Geometry check sheet. Reference: the model listing, model coordinates, mm. Face numbers are marked on the shaded views. A direction names the side the tool comes from. Coordinates: 2 decimals unless noted, no trailing zeros. Order: outer loops, then holes, each group sorted by start corner. A loop starts at its lowest first (then second) coordinate and runs counter-clockwise, first axis right, second up. Notation, with made-up numbers: (70, -39.5) - (100, -39.5) arc R34 ccw to (100, -1.5) - close; hole circle Ø5 at (-27, 22.5). An arc over 180 degrees is marked (long way). Use CSV: the item, a comma, the result in double quotes. Start each with the question number.
1) Sectioned sample at B-B, the plane z = 48. Record the cut outline in (x, y), and give its area (3 significant figures).
2) Thickness scan on probe 1 along X at (y, z) = (-7.25, 23.5); probe 2 along Z at (x, y) = (42, -3); probe 3 along Y at (x, z) = (40, -50). Record the ranges inside material, lowest first. Write a range as [from, to].
3) Tool access check on the marked faces 5 and 6. Record the directions out of +Z, -Z, +X, -X, +Y, -Y that give a thin tool (end or side, any length) a straight path to the whole face; none if there is none.
4) Sectioned sample at D-D, the plane x = 10. Record the cut outline in (y, z).
5) Sectioned sample at A-A, the plane z = 0. Record the cut outline in (x, y).
6) Depth check by flat-ended pin: P1, Ø1.1, axis at x = -38.5, y = -6.5, coming from the +Z side; P2, Ø5, axis at x = 6, y = -1.5, coming from the +Z side; P3, Ø1.3, axis at y = 1.5, z = -50, coming from the -X side; P4, Ø1.8, axis at y = 1.5, z = -50, coming from the +X side. Enter the tip coordinate at first touch or a pass-through.
7) Sectioned sample at C-C, the plane z = 24. Record the cut outline in (x, y), and give its area (3 significant figures).
8) Draft check along X on the marked faces 1, 2, 3 and 4. Enter one of: released by +X, released by -X, zero draft, split by the parting line, or undercut.
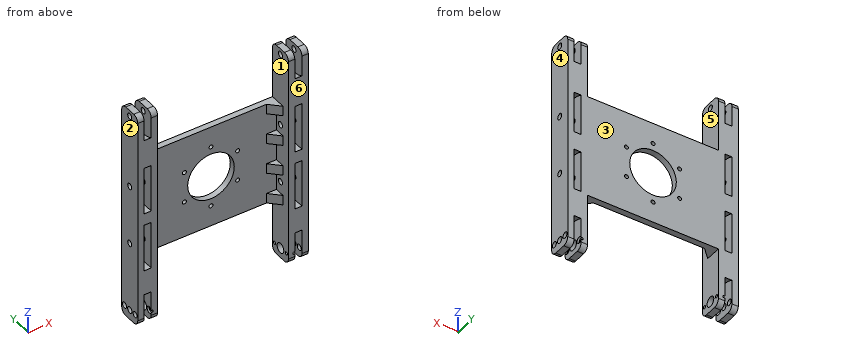
from build123d import *

# Parameters (mm, degrees)
SKETCH_1_W               = 66
SKETCH_1_H               = 52
EXTRUDE_1_DEPTH          = 3
SKETCH_2_W               = 110
SKETCH_2_H               = 12
EXTRUDE_2_DEPTH          = 10
CUT_EXTRUDE_1_REACH      = 96.244
SKETCH_4_R               = 1.6
SKETCH_4_R_2             = 1.5
SKETCH_8_R               = 12
CUT_EXTRUDE_4_DEPTH      = 1.8
CUT_EXTRUDE_2_REACH      = 88.383
SKETCH_5_R               = 0.8
SKETCH_5_R_2             = 2.5
CUT_EXTRUDE_5_REACH      = 96.244
SKETCH_10_R              = 1.5
SKETCH_11_R              = 1.6
CUT_EXTRUDE_6_DEPTH      = 1
FILLET_1_R               = 3
CUT_EXTRUDE_3_REACH      = 72.838
SKETCH_6_R               = 1
SKETCH_6_R_2             = 11.75
PATTERN_CIRCULAR_1_COUNT = 6
EXTRUDE_3_DEPTH          = 5
PATTERN_LINEAR_1_COUNT   = 4
PATTERN_LINEAR_1_PITCH   = 15.666666667
MIRROR_2_COPY_1_DEPTH    = 5
MIRROR_2_COPY_2_DEPTH    = 5
MIRROR_2_COPY_3_DEPTH    = 5


with BuildPart() as part:
    # Sketch 1 → Extrude 1 (new body)
    with BuildSketch(Plane(origin=(0, 0, 0), x_dir=(1, 0, 0), z_dir=(0, 1, 0))):
        Rectangle(SKETCH_1_W, SKETCH_1_H)
    extrude(amount=EXTRUDE_1_DEPTH)

    # Sketch 2 → Extrude 2 (add)
    with BuildSketch(Plane.ZY.offset(33)):
        with Locations((0, -3)):
            Rectangle(SKETCH_2_W, SKETCH_2_H)
    extrude_2 = extrude(amount=EXTRUDE_2_DEPTH)

    # Sketch 4 → Cut-Extrude 1 (cut, up to next)
    with BuildSketch(Plane.ZY.offset(43), mode=Mode.PRIVATE) as cut_extrude_1_sk1:
        with Locations((-50, -3)):
            Circle(SKETCH_4_R)
    cut_extrude_1_tool1 = extrude(cut_extrude_1_sk1.sketch, amount=-CUT_EXTRUDE_1_REACH, mode=Mode.PRIVATE) & part.part
    # Sketch 4 → Cut-Extrude 1 (cut, up to next)
    with BuildSketch(Plane.ZY.offset(43), mode=Mode.PRIVATE) as cut_extrude_1_sk2:
        with Locations((52, -3)):
            Circle(SKETCH_4_R_2)
    cut_extrude_1_tool2 = extrude(cut_extrude_1_sk2.sketch, amount=-CUT_EXTRUDE_1_REACH, mode=Mode.PRIVATE) & part.part
    # Sketch 4 → Cut-Extrude 1 (cut, up to next)
    with BuildSketch(Plane.ZY.offset(43), mode=Mode.PRIVATE) as cut_extrude_1_sk3:
        with Locations((-15, -3)):
            Circle(SKETCH_4_R_2)
    cut_extrude_1_tool3 = extrude(cut_extrude_1_sk3.sketch, amount=-CUT_EXTRUDE_1_REACH, mode=Mode.PRIVATE) & part.part
    # Sketch 4 → Cut-Extrude 1 (cut, up to next)
    with BuildSketch(Plane.ZY.offset(43), mode=Mode.PRIVATE) as cut_extrude_1_sk4:
        with Locations((15, -3)):
            Circle(SKETCH_4_R_2)
    cut_extrude_1_tool4 = extrude(cut_extrude_1_sk4.sketch, amount=-CUT_EXTRUDE_1_REACH, mode=Mode.PRIVATE) & part.part
    cut_extrude_1_1 = cut_extrude_1_tool1.solids().sort_by_distance((-43, -3, -50))[0]
    add(cut_extrude_1_1, mode=Mode.SUBTRACT)
    cut_extrude_1_2 = cut_extrude_1_tool2.solids().sort_by_distance((-43, -3, 52))[0]
    add(cut_extrude_1_2, mode=Mode.SUBTRACT)
    cut_extrude_1_3 = cut_extrude_1_tool3.solids().sort_by_distance((-43, -3, -15))[0]
    add(cut_extrude_1_3, mode=Mode.SUBTRACT)
    cut_extrude_1_4 = cut_extrude_1_tool4.solids().sort_by_distance((-43, -3, 15))[0]
    add(cut_extrude_1_4, mode=Mode.SUBTRACT)
    cut_extrude_1 = cut_extrude_1_1 + cut_extrude_1_2 + cut_extrude_1_3 + cut_extrude_1_4  # Cut-Extrude 1 as one shape, for the pattern or mirror that repeats it

    # Sketch 8 → Cut-Extrude 4 (cut, symmetric)
    with BuildSketch(Plane(origin=(-38, 0, 0), x_dir=(0, 0, -1), z_dir=(1, 0, 0))):
        with Locations((-52, -3)):
            Circle(SKETCH_8_R)
        with Locations((50, -3)):
            Circle(SKETCH_8_R)
        with BuildLine():
            Line((-27, -3), (-27, -9))
            Line((-27, -9), (-3, -9))
            Line((-3, -9), (-3, -3))
            ThreePointArc((-3, -3), (-15, 9), (-27, -3))
        make_face()
        with BuildLine():
            Line((3, -3), (3, -9))
            Line((3, -9), (27, -9))
            Line((27, -9), (27, -3))
            ThreePointArc((27, -3), (15, 9), (3, -3))
        make_face()
    cut_extrude_4 = extrude(amount=CUT_EXTRUDE_4_DEPTH, both=True, mode=Mode.SUBTRACT)

    # Sketch 5 → Cut-Extrude 2 (cut, up to next)
    with BuildSketch(Plane.ZY.offset(33), mode=Mode.PRIVATE) as cut_extrude_2_sk1:
        with Locations(Location((-50, 1.5, 0), (0, 0, 180))):
            Circle(SKETCH_5_R)
    cut_extrude_2_tool1 = extrude(cut_extrude_2_sk1.sketch, amount=CUT_EXTRUDE_2_REACH, mode=Mode.PRIVATE) & part.part
    # Sketch 5 → Cut-Extrude 2 (cut, up to next)
    with BuildSketch(Plane.ZY.offset(33), mode=Mode.PRIVATE) as cut_extrude_2_sk2:
        with Locations(Location((-50, -7.5, 0), (0, 0, 180))):
            Circle(SKETCH_5_R)
    cut_extrude_2_tool2 = extrude(cut_extrude_2_sk2.sketch, amount=CUT_EXTRUDE_2_REACH, mode=Mode.PRIVATE) & part.part
    # Sketch 5 → Cut-Extrude 2 (cut, up to next)
    with BuildSketch(Plane.ZY.offset(33), mode=Mode.PRIVATE) as cut_extrude_2_sk3:
        with Locations(Location((-50, -3, 0), (0, 0, 180))):
            Circle(SKETCH_5_R_2)
    cut_extrude_2_tool3 = extrude(cut_extrude_2_sk3.sketch, amount=CUT_EXTRUDE_2_REACH, mode=Mode.PRIVATE) & part.part
    cut_extrude_2_1 = cut_extrude_2_tool1.solids().sort_by_distance((-33, 1.5, -50))[0]
    add(cut_extrude_2_1, mode=Mode.SUBTRACT)
    cut_extrude_2_2 = cut_extrude_2_tool2.solids().sort_by_distance((-33, -7.5, -50))[0]
    add(cut_extrude_2_2, mode=Mode.SUBTRACT)
    cut_extrude_2_3 = cut_extrude_2_tool3.solids().sort_by_distance((-33, -3, -50))[0]
    add(cut_extrude_2_3, mode=Mode.SUBTRACT)
    cut_extrude_2 = cut_extrude_2_1 + cut_extrude_2_2 + cut_extrude_2_3  # Cut-Extrude 2 as one shape, for the pattern or mirror that repeats it

    # Sketch 10 → Cut-Extrude 5 (cut, up to next)
    with BuildSketch(Plane.ZY.offset(43), mode=Mode.PRIVATE) as cut_extrude_5_sk1:
        with Locations((-50, -7)):
            Circle(SKETCH_10_R)
    cut_extrude_5_tool1 = extrude(cut_extrude_5_sk1.sketch, amount=-CUT_EXTRUDE_5_REACH, mode=Mode.PRIVATE) & part.part
    # Sketch 10 → Cut-Extrude 5 (cut, up to next)
    with BuildSketch(Plane.ZY.offset(43), mode=Mode.PRIVATE) as cut_extrude_5_sk2:
        with Locations((-50, 1)):
            Circle(SKETCH_10_R)
    cut_extrude_5_tool2 = extrude(cut_extrude_5_sk2.sketch, amount=-CUT_EXTRUDE_5_REACH, mode=Mode.PRIVATE) & part.part
    cut_extrude_5_1 = cut_extrude_5_tool1.solids().sort_by_distance((-43, -7, -50))[0]
    add(cut_extrude_5_1, mode=Mode.SUBTRACT)
    cut_extrude_5_2 = cut_extrude_5_tool2.solids().sort_by_distance((-43, 1, -50))[0]
    add(cut_extrude_5_2, mode=Mode.SUBTRACT)
    cut_extrude_5 = cut_extrude_5_1 + cut_extrude_5_2  # Cut-Extrude 5 as one shape, for the pattern or mirror that repeats it

    # Sketch 11 → Cut-Extrude 6 (cut)
    with BuildSketch(Plane.ZY.offset(36.2)):
        with Locations((-50, 1.5)):
            Circle(SKETCH_11_R)
        with Locations((-50, -7.5)):
            Circle(SKETCH_11_R)
    cut_extrude_6 = extrude(amount=-CUT_EXTRUDE_6_DEPTH, mode=Mode.SUBTRACT)

    # Mirror 1: Extrude 2, Cut-Extrude 1, Cut-Extrude 4, Cut-Extrude 2, Cut-Extrude 5, Cut-Extrude 6 across plane
    add(extrude_2.mirror(Plane(origin=(0, 0, 0), x_dir=(0, 0, 1), z_dir=(1, 0, 0))))
    add(cut_extrude_1.mirror(Plane(origin=(0, 0, 0), x_dir=(0, 0, 1), z_dir=(1, 0, 0))), mode=Mode.SUBTRACT)
    add(cut_extrude_4.mirror(Plane(origin=(0, 0, 0), x_dir=(0, 0, 1), z_dir=(1, 0, 0))), mode=Mode.SUBTRACT)
    add(cut_extrude_2.mirror(Plane(origin=(0, 0, 0), x_dir=(0, 0, 1), z_dir=(1, 0, 0))), mode=Mode.SUBTRACT)
    add(cut_extrude_5.mirror(Plane(origin=(0, 0, 0), x_dir=(0, 0, 1), z_dir=(1, 0, 0))), mode=Mode.SUBTRACT)
    add(cut_extrude_6.mirror(Plane(origin=(0, 0, 0), x_dir=(0, 0, 1), z_dir=(1, 0, 0))), mode=Mode.SUBTRACT)

    # Fillet 1
    fillet_1_edges = [part.edges().sort_by_distance(p)[0] for p in [
        (-41.4, 3, -55),
        (-41.4, -9, -55),
        (-41.4, -9, 55),
        (-41.4, 3, 55),
        (41.4, -9, -55),
        (41.4, 3, -55),
        (41.4, 3, 55),
        (41.4, -9, 55),
        (34.6, -9, 55),
        (34.6, 3, 55),
        (34.6, -9, -55),
        (34.6, 3, -55),
        (-34.6, 3, 55),
        (-34.6, -9, 55),
        (-34.6, -9, -55),
        (-34.6, 3, -55),
    ]]
    fillet(fillet_1_edges, radius=FILLET_1_R)

    # Sketch 6 → Cut-Extrude 3 (cut, up to next)
    with BuildSketch(Plane(origin=(0, 3, 0), x_dir=(1, 0, 0), z_dir=(0, 1, 0)), mode=Mode.PRIVATE) as cut_extrude_3_sk1:
        with Locations(Location((0, 15.5, 0), (0, 0, 270))):
            Circle(SKETCH_6_R)
    cut_extrude_3_tool1 = extrude(cut_extrude_3_sk1.sketch, amount=-CUT_EXTRUDE_3_REACH, mode=Mode.PRIVATE) & part.part
    # Sketch 6 → Cut-Extrude 3 (cut, up to next)
    with BuildSketch(Plane(origin=(0, 3, 0), x_dir=(1, 0, 0), z_dir=(0, 1, 0)), mode=Mode.PRIVATE) as cut_extrude_3_sk2:
        with Locations(Location((0, 0, 0), (0, 0, 270))):
            Circle(SKETCH_6_R_2)
    cut_extrude_3_tool2 = extrude(cut_extrude_3_sk2.sketch, amount=-CUT_EXTRUDE_3_REACH, mode=Mode.PRIVATE) & part.part
    cut_extrude_3_1 = cut_extrude_3_tool1.solids().sort_by_distance((0, 3, -15.5))[0]
    add(cut_extrude_3_1, mode=Mode.SUBTRACT)
    cut_extrude_3_2 = cut_extrude_3_tool2.solids().sort_by_distance((0, 3, 0))[0]
    add(cut_extrude_3_2, mode=Mode.SUBTRACT)
    cut_extrude_3 = cut_extrude_3_1 + cut_extrude_3_2  # Cut-Extrude 3 as one shape, for the pattern or mirror that repeats it

    # Pattern Circular 1: Cut-Extrude 3 ×6 about axis
    pattern_circular_1_axis = Axis((0, 0, 0), (0, 1, 0))
    for i in range(1, PATTERN_CIRCULAR_1_COUNT):
        add(cut_extrude_3.rotate(pattern_circular_1_axis, i * 360 / PATTERN_CIRCULAR_1_COUNT), mode=Mode.SUBTRACT)

    # Sketch 9 → Extrude 3 (add)
    with BuildSketch(Plane(origin=(0, 0, -26), x_dir=(-1, 0, 0), z_dir=(0, 0, -1))):
        Polygon((33, 0), (28, 0), (33, -5), align=None)
    extrude_3 = extrude(amount=-EXTRUDE_3_DEPTH)

    # Pattern Linear 1: Extrude 3 ×4
    with Locations(*[(0, 0, i * PATTERN_LINEAR_1_PITCH) for i in range(1, PATTERN_LINEAR_1_COUNT)]):
        add(extrude_3)

    # Mirror 2: Extrude 3 across plane
    add(extrude_3.mirror(Plane(origin=(0, 0, 0), x_dir=(0, 0, 1), z_dir=(1, 0, 0))))

    # Mirror 2 copy 1 sketch → Mirror 2 copy 1 (add)
    with BuildSketch(Plane(origin=(0, 0, -10.333333333), x_dir=(1, 0, 0), z_dir=(0, 0, -1))):
        Polygon((33, 0), (28, 0), (33, 5), align=None)
    extrude(amount=-MIRROR_2_COPY_1_DEPTH)

    # Mirror 2 copy 2 sketch → Mirror 2 copy 2 (add)
    with BuildSketch(Plane(origin=(0, 0, 5.333333333), x_dir=(1, 0, 0), z_dir=(0, 0, -1))):
        Polygon((33, 0), (28, 0), (33, 5), align=None)
    extrude(amount=-MIRROR_2_COPY_2_DEPTH)

    # Mirror 2 copy 3 sketch → Mirror 2 copy 3 (add)
    with BuildSketch(Plane(origin=(0, 0, 21), x_dir=(1, 0, 0), z_dir=(0, 0, -1))):
        Polygon((33, 0), (28, 0), (33, 5), align=None)
    extrude(amount=-MIRROR_2_COPY_3_DEPTH)


solid = part.part
Evaluation:
1,outline,"(-43, -9) - (-39.8, -9) - (-39.8, 3) - (-43, 3) - close; (-36.2, -9) - (-33, -9) - (-33, 3) - (-36.2, 3) - close; (33, -9) - (36.2, -9) - (36.2, 3) - (33, 3) - close; (39.8, -9) - (43, -9) - (43, 3) - (39.8, 3) - close"
1,area,"154 mm²"
2,probe 1,"[-43, -39.8], [-36.2, -33], [33, 36.2], [39.8, 43]"
2,probe 2,"[-55, -51.6], [-48.4, -16.5], [-13.5, 13.5], [16.5, 50.5], [53.5, 55]"
2,probe 3,"[-9, -8.5], [-5.5, -4.6], [-1.4, -0.5], [2.5, 3]"
3,face 5,"-Y"
3,face 6,"+Z, -Z, +X, -X, -Y"
4,outline,"(0, -26) - (3, -26) - (3, -6.17) - (0, -6.17) - close; (0, 6.17) - (3, 6.17) - (3, 26) - (0, 26) - close"
5,outline,"(-43, -9) - (-33, -9) - (-33, 0) - (-11.75, 0) - (-11.75, 3) - (-43, 3) - close; (11.75, 0) - (33, 0) - (33, -9) - (43, -9) - (43, 3) - (11.75, 3) - close"
6,P1,"z = 40.7"
6,P2,"z = 26"
6,P3,"through"
6,P4,"x = 35.2"
7,outline,"(-43, -9) - (-39.8, -9) - (-39.8, 3) - (-43, 3) - close; (-36.2, -9) - (-33, -9) - (-33, -5) - (-28, 0) - (28, 0) - (33, -5) - (33, -9) - (36.2, -9) - (36.2, 3) - (-36.2, 3) - close; (39.8, -9) - (43, -9) - (43, 3) - (39.8, 3) - close"
7,area,"377 mm²"
8,face 1,"undercut"
8,face 2,"released by -X"
8,face 3,"zero draft"
8,face 4,"released by +X"
